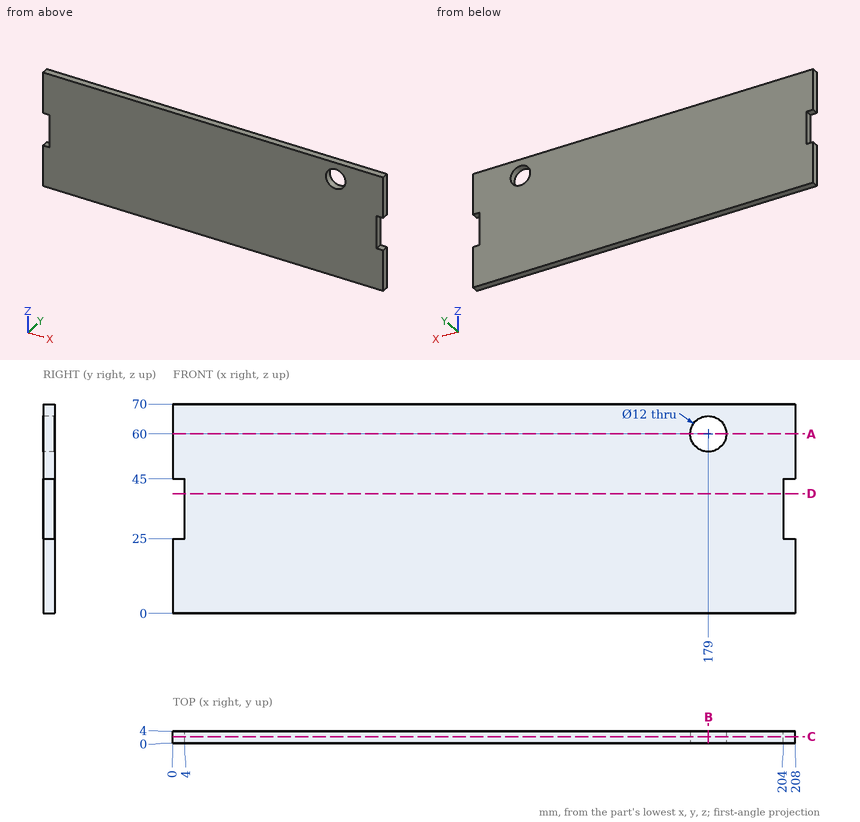
Print and shaded views of the part. All mm, measured from the part's lowest x, y and z. Round coordinates to 2 decimals unless told otherwise and drop trailing zeros. Write each loop counter-clockwise with the first axis right and the second up, starting at its lowest first coordinate (ties: lowest second). Pieces come first, ordered by that corner, then holes.
(1) Slice it at B-B, the plane x = 179. Write the cut outline in (y, z).
(2) Slice it at D-D, the plane z = 40. Write the cut outline in (x, y).
(3) Slice it at A-A, the plane z = 60. Write the cut outline in (x, y).
(4) Slice it at C-C, the plane y = 2.2. Write the cut outline in (x, z).
(5) Probe line 1 along X through (y, z) = (1.4, 60); line 2 along X through (y, z) = (0.5, 26); line 3 along X through (y, z) = (2.85, 58.5). List the from-to ranges inside material, lowest first.
(6) Drop a flat-ended pin along its axis: P1, Ø7, axis at x = 179, z = 60, coming from the -Y side. Give the stop position or say it passes through.
From the geometry:
1. outline: (0, 0) - (4, 0) - (4, 54) - (0, 54) - close; (0, 66) - (4, 66) - (4, 70) - (0, 70) - close
2. outline: (4, 0) - (204, 0) - (204, 4) - (4, 4) - close
3. outline: (0, 0) - (173, 0) - (173, 4) - (0, 4) - close; (185, 0) - (208, 0) - (208, 4) - (185, 4) - close
4. outline: (0, 0) - (208, 0) - (208, 25) - (204, 25) - (204, 45) - (208, 45) - (208, 70) - (0, 70) - (0, 45) - (4, 45) - (4, 25) - (0, 25) - close; hole circle Ø12 at (179, 60)
5. line 1: x = 0 to 173, 185 to 208
5. line 2: x = 4 to 204
5. line 3: x = 0 to 173.19, 184.81 to 208
6. P1: passes through
